Solid Edge part; units mm, degrees
sketch "Sketch1" plane through (0, 0, 0) normal (0, -1, 0) x (1, 0, 0)
  line L0 (15, 28) -> (15, -28)
  line L1 (15, -28) -> (-15, -28)
  line L2 (-15, -28) -> (-15, 28)
  line L3 (-15, 28) -> (15, 28)
  line L4 (10.1, 20.5) -> (10.1, -20.5)
  line L5 (10.1, -20.5) -> (-10.1, -20.5)
  line L6 (-10.1, -20.5) -> (-10.1, 20.5)
  line L7 (-10.1, 20.5) -> (10.1, 20.5)
extrude "Protrusion1" add sketch "Sketch1" along normal mid plane 10
Verification items for the finished model (mm, model axes). A direction names the side the tool comes from. Coordinates: 2 decimals unless noted, no trailing zeros. Loops run counter-clockwise (first coordinate to the right, second up) from the corner with the lowest first, then second, coordinate; pieces in that order, holes last. Notation, with made-up numbers: (29.5, 56.25) -> (52.5, 56.25) arc R13 ccw to (52.5, 60.25) -> close; hole circle Ø9 at (-4.5, 32). An arc over 180 degrees is marked (long way). Put each result on its own line as item: value.
1. Section check A-A, the plane z = -3. Record the boundary of the cut face in (x, y), then the cut area to 3 significant figures.
Result set:
outline: (-15, -5) -> (-10.1, -5) -> (-10.1, 5) -> (-15, 5) -> close; (10.1, -5) -> (15, -5) -> (15, 5) -> (10.1, 5) -> close
area: 98.0 mm^2
2. Thickness scan on line 1 (Z direction, x = -3.75, y = 4); line 2 (X direction, y = 4.75, z = -19.5). Record the ranges inside material, lowest first.
Result set:
line 1: z = -28 to -20.5, 20.5 to 28
line 2: x = -15 to -10.1, 10.1 to 15
3. Tool access check on faces 1 (the face through (14, 5, 0)), 2 (the face through (0, 0, -20.5)). Record the directions out of +Z, -Z, +X, -X, +Y, -Y that give a thin tool (end or side, any length) a straight path to the whole face; none if there is none.
Result set:
face 1: +Z, -Z, +X, -X, +Y
face 2: +Y, -Y
4. Mould release check, pull along Z, two halves, no side actions. Record for faces 3 (the face through (15, 0, 0)), 4 (the face through (0, 0, 20.5)), 5 (the face through (10.1, 0, 0)), 6 (the face through (0, 0, 28)): pulls with the +Z half, pulls with the -Z half, needs draft (parallel to the pull), parting line crosses it, or undercut.
Result set:
face 3: needs draft
face 4: undercut
face 5: undercut
face 6: pulls with the +Z half
5. Section check C-C, the plane y = -3.5. Record the boundary of the cut face in (x, z), then the cut area to 3 significant figures.
Result set:
outline: (-15, -28) -> (15, -28) -> (15, 28) -> (-15, 28) -> close; hole (-10.1, -20.5) -> (10.1, -20.5) -> (10.1, 20.5) -> (-10.1, 20.5) -> close
area: 852 mm^2
6. Section check B-B, the plane x = 1.75. Record the boundary of the cut face in (y, z).
Result set:
outline: (-5, -28) -> (5, -28) -> (5, -20.5) -> (-5, -20.5) -> close; (-5, 20.5) -> (5, 20.5) -> (5, 28) -> (-5, 28) -> close
